Check sheet for the modelled part. Datum: model origin and axes. Units: mm. A direction names the side the tool comes from. Give positions to 0.01 mm unless a question says otherwise; leave off trailing zeros. Order: outer loops, then holes, each group sorted by start corner. A loop starts at its lowest first (then second) coordinate and runs counter-clockwise, first axis right, second up. Notation, with made-up numbers: (37.25, 85) -> (79.25, 85) arc R16 cw to (79.25, 100) -> close; hole circle Ø7 at (48, 23.25). An arc over 180 degrees is marked (long way). Answer in a Markdown table with one row per item. Add a question column.
(1) Release check for a two-part mould opening along Z. For faces 1 (the face through (26.5, -67, 5)), 2 (the face through (18, -133, 5)), 3 (the face through (22, -66, 0)) record: released by +Z, released by -Z, zero draft, split by the parting line, or undercut.
(2) Cross-section at C-C (y = -128). Record the cut outline in (x, z).
(3) Cross-section at A-A (z = 5). Record the cut outline in (x, y), then the cut area to 3 significant figures.
(4) Go/stop test with a flat-tipped pin: pin 1 (2.5 mm diameter, centred on y = -15, z = 5, fed in from -X). Record where the tip stops, or that it passes through.
(5) Set-up check for faces 4 (the face through (18.5, -67, 5)), 5 (the face through (27.007, -116.474, 5.481)): record each of +Z, -Z, +X, -X, +Y, -Y from which the full face is reachable in a straight line by a thin tool's end or side.
(6) Cross-section at B-B (y = -32.5). Record the cut outline in (x, z), then the cut area to 3 significant figures.
(7) Thickness scan on L1, parallel to Y at x = 27, z = 5.25; L2, parallel to Z at x = 22.5, y = -117; L3, parallel to X at y = -5, z = 9.3. Record the ranges inside material, lowest first. Write a range as [from, to].
```python
from build123d import *

# Parameters (mm, degrees)
SKETCH_1_W          = 10
SKETCH_1_H          = 133
SKETCH_1_R          = 1.6
EXTRUDE_1_DEPTH     = 10
SKETCH_2_R          = 1.6
CUT_EXTRUDE_1_DEPTH = 15
SKETCH_3_W          = 8
SKETCH_3_H          = 8
CUT_EXTRUDE_2_DEPTH = 1000


with BuildPart() as part:
    # ｽｹｯﾁ1 → ﾎﾞｽ - 押し出し1 (new body)
    with BuildSketch(Plane.XY):
        with Locations((22.499828612, -66.5)):
            Rectangle(SKETCH_1_W, SKETCH_1_H)
        with Locations((22.499828612, -5)):
            Circle(SKETCH_1_R, mode=Mode.SUBTRACT)
        with Locations((22.499828612, -128)):
            Circle(SKETCH_1_R, mode=Mode.SUBTRACT)
    extrude(amount=EXTRUDE_1_DEPTH)

    # ｽｹｯﾁ2 → ｶｯﾄ - 押し出し1 (cut)
    with BuildSketch(Plane(origin=(27.499828612, 0, 0), x_dir=(0, 0, -1), z_dir=(1, 0, 0))):
        with Locations(Location((-5, -118, 0), (0, 0, 90))):
            Circle(SKETCH_2_R)
        with Locations(Location((-5, -15, 0), (0, 0, 90))):
            Circle(SKETCH_2_R)
    extrude(amount=-CUT_EXTRUDE_1_DEPTH, mode=Mode.SUBTRACT)

    # ｽｹｯﾁ3 → ｶｯﾄ - 押し出し2 (cut)
    with BuildSketch(Plane.XZ.offset(133)):
        with Locations((22.499828612, 5)):
            Rectangle(SKETCH_3_W, SKETCH_3_H)
    extrude(amount=-CUT_EXTRUDE_2_DEPTH, mode=Mode.SUBTRACT)


solid = part.part
```
Answer below:
| question | item | result |
|---|---|---|
| 1 | face 1 | undercut |
| 1 | face 2 | zero draft |
| 1 | face 3 | released by -Z |
| 2 | outline | (17.5, 0) -> (20.9, 0) -> (20.9, 1) -> (18.5, 1) -> (18.5, 9) -> (20.9, 9) -> (20.9, 10) -> (17.5, 10) -> close; (24.1, 0) -> (27.5, 0) -> (27.5, 10) -> (24.1, 10) -> (24.1, 9) -> (26.5, 9) -> (26.5, 1) -> (24.1, 1) -> close |
| 3 | outline | (17.5, -133) -> (18.5, -133) -> (18.5, -119.6) -> (17.5, -119.6) -> close; (17.5, -116.4) -> (18.5, -116.4) -> (18.5, -16.6) -> (17.5, -16.6) -> close; (17.5, -13.4) -> (18.5, -13.4) -> (18.5, 0) -> (17.5, 0) -> close; (26.5, -133) -> (27.5, -133) -> (27.5, -119.6) -> (26.5, -119.6) -> close; (26.5, -116.4) -> (27.5, -116.4) -> (27.5, -16.6) -> (26.5, -16.6) -> close; (26.5, -13.4) -> (27.5, -13.4) -> (27.5, 0) -> (26.5, 0) -> close |
| 3 | area | 253 mm² |
| 4 | pin 1 | passes through |
| 5 | face 4 | +Y, -Y |
| 5 | face 5 | +X, -X |
| 6 | outline | (17.5, 0) -> (27.5, 0) -> (27.5, 10) -> (17.5, 10) -> close; hole (18.5, 1) -> (26.5, 1) -> (26.5, 9) -> (18.5, 9) -> close |
| 6 | area | 36.0 mm² |
| 7 | L1 | y = [-133, -119.58], [-116.42, -16.58], [-13.42, 0] |
| 7 | L2 | z = [0, 1], [9, 10] |
| 7 | L3 | x = [17.5, 20.9], [24.1, 27.5] |
